Verification items for the finished model (mm, model axes). Coordinates: 2 decimals unless noted, no trailing zeros. Order: outer loops, then holes, each group sorted by start corner. A loop starts at its lowest first (then second) coordinate and runs counter-clockwise, first axis right, second up. Notation, with made-up numbers: (-25.75, 24.25) - (-18.75, 24.25) arc R21 cw to (-18.75, 50.25) - close; hole circle Ø2 at (-33, 71.5). An arc over 180 degrees is marked (long way). Answer as CSV lines item,"result". Start each with the question number.
1. Section check C-C (z = 2.75). Count the separate pieces of the cut face and the enclosed holes in it, and give its area (3 significant figures).
2. Material ranges on L1, parallel to Y at x = 63.5, z = 1.5; L2, parallel to X at y = 36, z = 5.5; L3, parallel to X at y = 75.5, z = 1.75, recorded low to high. Write a range as [from, to].
3. Section check D-D (x = 63.5). Record the cut outline in (y, z).
4. Section check A-A (x = 12.7). Record the cut outline in (y, z).
5. Go/stop test with flat-tipped pins: pin 1 (2 mm diameter, centred on y = 84, z = 1, fed in from +X); pin 2 (6 mm diameter, centred on x = 63.5, y = 63.5, fed in from -Z); pin 3 (1.5 mm diameter, centred on y = 51, z = 3, fed in from -X). Record where each tip stops, or that it passes through.
6. Mould release check, pull along Y, two halves, no side actions. Record for faces 1 (the flat face through (127, 13, 3)), 2 (the cylindrical face through (63.077, 34.876, 3.131)), 3 (the flat face through (64, 101.6, 3)), 4 (the cylindrical face through (39.6, 66.384, 3.131)): pulls with the +Y half, pulls with the -Y half, needs draft (parallel to the pull), parting line crosses it, or undercut.
7. Section check B-B (y = 63.5). Record the cut outline in (x, z).
Autodesk Inventor part; units mm, degrees
ref_plane "YZ Plane" through (0, 0, 0) normal (1, 0, 0) x (0, 1, 0)
ref_plane "XZ Plane" through (0, 0, 0) normal (0, 1, 0) x (-1, 0, 0)
ref_plane "XY Plane" through (0, 0, 0) normal (0, 0, 1) x (1, 0, 0)
sketch "Sketch1" plane through (0, 0, 0) normal (0, 0, 1) x (1, 0, 0)
  line L0 (0, 0) -> (127, 0)
  line L1 (127, 0) -> (127, 101.6)
  line L2 (101.6, 101.6) -> (0, 101.6)
  line L3 (0, 25.4) -> (0, 0)
  circle A0 centre (12.7, 12.7) radius 3.2512
  circle A1 centre (38.1, 12.7) radius 3.2512
  circle A2 centre (63.5, 12.7) radius 3.2512
  circle A3 centre (88.9, 12.7) radius 3.2512
  circle A4 centre (114.3, 12.7) radius 3.2512
  circle A5 centre (38.1, 38.1) radius 3.2512
  circle A6 centre (63.5, 38.1) radius 3.2512
  circle A7 centre (88.9, 38.1) radius 3.2512
  circle A8 centre (38.1, 63.5) radius 3.2512
  circle A9 centre (63.5, 63.5) radius 3.2512
  circle A10 centre (88.9, 63.5) radius 3.2512
  circle A11 centre (38.1, 88.9) radius 3.2512
  circle A12 centre (63.5, 88.9) radius 3.2512
  circle A13 centre (88.9, 88.9) radius 3.2512
  line L4 (0, 25.4) -> (25.4, 101.6)
  line L5 (101.6, 101.6) -> (127, 25.4)
  dimension "d2" = 127
  dimension "d3" = 101.6
  dimension "d4" = 6.5024
  dimension "d5" = 12.7
  dimension "d6" = 12.7
  dimension "d9" = 25.4
  dimension "d14" = 25.4
  dimension "d15" = 25.4
  dimension "d18" = 25.4
  dimension "d23" = 25.4
  dimension "d24" = 25.4
extrude "Extrusion1" add sketch "Sketch1" along normal blind 6.35
properties part number "3x1 T plate"
Evaluation:
1,separate pieces,"1"
1,enclosed holes,"14"
1,area,"10,500 mm²"
2,L1,"y = [0, 9.45], [15.95, 34.85], [41.35, 60.25], [66.75, 85.65], [92.15, 101.6]"
2,L2,"x = [3.53, 35.62], [40.58, 61.02], [65.98, 86.42], [91.38, 123.47]"
2,L3,"x = [16.7, 110.3]"
3,outline,"(0, 0) - (9.45, 0) - (9.45, 6.35) - (0, 6.35) - close; (15.95, 0) - (34.85, 0) - (34.85, 6.35) - (15.95, 6.35) - close; (41.35, 0) - (60.25, 0) - (60.25, 6.35) - (41.35, 6.35) - close; (66.75, 0) - (85.65, 0) - (85.65, 6.35) - (66.75, 6.35) - close; (92.15, 0) - (101.6, 0) - (101.6, 6.35) - (92.15, 6.35) - close"
4,outline,"(0, 0) - (9.45, 0) - (9.45, 6.35) - (0, 6.35) - close; (15.95, 0) - (63.5, 0) - (63.5, 6.35) - (15.95, 6.35) - close"
5,pin 1,"stops at x = 107.8"
5,pin 2,"passes through"
5,pin 3,"stops at x = 8.28"
6,face 1,"needs draft"
6,face 2,"undercut"
6,face 3,"pulls with the +Y half"
6,face 4,"undercut"
7,outline,"(12.7, 0) - (34.85, 0) - (34.85, 6.35) - (12.7, 6.35) - close; (41.35, 0) - (60.25, 0) - (60.25, 6.35) - (41.35, 6.35) - close; (66.75, 0) - (85.65, 0) - (85.65, 6.35) - (66.75, 6.35) - close; (92.15, 0) - (114.3, 0) - (114.3, 6.35) - (92.15, 6.35) - close"
